Autodesk Inventor part; units mm, degrees
ref_plane "Work Plane2" through (46, 0, 28.75) normal (0.8365, -0.5, 0.2241) x (-0.2588, 0, 0.9659)
ref_plane "YZ Plane" through (0, 0, 0) normal (1, 0, 0) x (0, 1, 0)
ref_plane "XZ Plane" through (0, 0, 0) normal (0, 1, 0) x (-1, 0, 0)
sketch "Sketch1" plane through (0, 0, 0) normal (0, 0, 1) x (1, 0, 0)
  circle A0 centre (0, 0) radius 5
  circle A1 centre (0, 0) radius 8.45
  circle A2 centre (0, 0) radius 42.5
  circle A3 centre (0, 0) radius 45 construction
  circle A4 centre (-31.8198, 31.8198) radius 1.45
  arc A5 (-28.0933, 35.1535) -> (-35.1535, 28.0933) centre (-31.8198, 31.8198) ccw
  arc A6 (-35.1535, -28.0933) -> (-28.0933, -35.1535) centre (-31.8198, -31.8198) ccw
  circle A7 centre (-31.8198, -31.8198) radius 1.45
  arc A8 (28.0933, -35.1535) -> (35.1535, -28.0933) centre (31.8198, -31.8198) ccw
  circle A9 centre (31.8198, -31.8198) radius 1.45
  arc A10 (35.1535, 28.0933) -> (28.0933, 35.1535) centre (31.8198, 31.8198) ccw
  circle A11 centre (31.8198, 31.8198) radius 1.45
  line L0 (-31.8198, 31.8198) -> (31.8198, 31.8198) construction
  arc A12 (28.841, 35.8357) -> (-28.841, 35.8357) centre (0, 0) ccw
  arc A13 (-35.8357, 28.841) -> (-35.8357, -28.841) centre (0, 0) ccw
  arc A14 (-28.841, -35.8357) -> (28.841, -35.8357) centre (0, 0) ccw
  arc A15 (35.8357, -28.841) -> (35.8357, 28.841) centre (0, 0) ccw
  point P0 (0, -46)
  point P1 (0, 46)
  dimension "d2" = 10
  dimension "d3" = 16.9
  dimension "d4" = 85
  dimension "d5" = 90
  dimension "d6" = 2.9
  dimension "d7" = 5
  dimension "d8" = 360
  dimension "d9" = 92
extrude "Extrusion1" add sketch "Sketch1" along normal blind 2.5 contours A1
extrude "Extrusion2" add sketch "Sketch1" along normal blind 7.5 contours A2
extrude "Extrusion3" add sketch "Sketch1" along normal blind 28.75 contours A12 A10 A15 A8 A14 A6 A13 A5
sketch "Sketch2" plane through (0, 0, 28.75) normal (0, 0, 1) x (1, 0, 0)
  arc A0 (35.8357, -28.841) -> (35.8357, 28.841) centre (0, 0) ccw construction
  line L0 (46, 0) -> (46, -31.8198) construction
  point P0 (31.8198, -31.8198)
ref_plane "Work Plane1" through (46, 0, 28.75) normal (0.9659, 0, 0.2588) x (0, -1, 0)
sketch "Sketch3" plane through (46, 0, 28.75) normal (0.9659, 0, 0.2588) x (0, -1, 0)
  ellipse E0 centre (0, -11.9057) end of major axis (-46, -11.9057) minor radius 11.9057 (28.841, -2.6307) -> (-28.841, -2.6307) ccw
  line L0 (0, 0) -> (0, -11.9057) construction
  point P0 (0, 15.8647)
ref_plane "Work Plane2" through (46, 0, 28.75) normal (0.8365, -0.5, 0.2241) x (-0.2588, 0, 0.9659)
sketch "Sketch4" plane through (46, 0, 28.75) normal (0.8365, -0.5, 0.2241) x (-0.2588, 0, 0.9659)
  circle A0 centre (0, 0) radius 5.325
  point P0 (-15.8647, 25.9368)
  dimension "d18" = 10.65
extrude "Extrusion4" cut sketch "Sketch4" along normal mid plane 30
properties part number "Case Part 1 - V2"
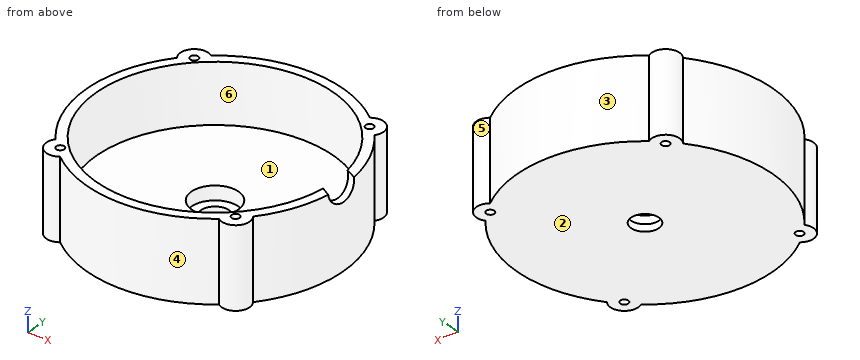
Could you check a few things on this model? Use its own coordinates, in mm. Face numbers are marked on the shaded views. A direction names the side the tool comes from. Give positions to 0.01 mm unless a question says otherwise; leave off trailing zeros. Order: outer loops, then holes, each group sorted by start corner. A loop starts at its lowest first (then second) coordinate and runs counter-clockwise, first axis right, second up.
1. For the marked faces 5 and 6, which set-ups out of +Z, -Z, +X, -X, +Y, -Y let a thin tool reach every point of the face, with its end or its side?
2. We'd pull the mould along Y, two halves only. Please class the marked faces 1, 2, 3 and 4: pulls with the +Y half, pulls with the -Y half, needs draft (parallel to the pull), parting line crosses it, or undercut.
3. I need wall thicknesses on L1, parallel to Y at x = -1, z = 9; L2, parallel to Y at x = 36, z = 19.5. Which ranges of each line are inside material? Lowest first, please.
4. Suppose I cut it at C-C (z = 13.25). List the corners of the cut face in (x, y) for me, plus the area to 3 significant figures.
5. Suppose I cut it at D-D (x = -27). List the corners of the cut face in (y, z) for me.
6. Suppose I cut it at B-B (y = -16.5). List the corners of the cut face in (x, z) for me.
7. Suppose I cut it at A-A (x = 0). List the corners of the cut face in (y, z) for me.
8. Will these pins go through, and if not, where does the flat tip stop? P1, Ø1.7, axis at x = -31.82, y = -31.82, coming from the -Z side; P2, Ø1.5, axis at y = -12, z = 13.5, coming from the +X side; P3, Ø2, axis at y = -28.5, z = 7.5, coming from the -X side; P4, Ø1.5, axis at x = 21.5, z = 22.5, coming from the +Y side.
Solved:
1. face 5: +Z, -Z
1. face 6: +Z
2. face 1: undercut
2. face 2: needs draft
2. face 3: pulls with the +Y half
2. face 4: pulls with the -Y half
3. L1: y = -45.99 to -42.49, 42.49 to 45.99
3. L2: y = -34.56 to -29.08, -28.64 to -22.59, 22.59 to 28.64, 29.08 to 34.56
4. outline: (-35.84, -28.84) arc R5 ccw to (-28.84, -35.84) arc R46 ccw to (28.84, -35.84) arc R5 ccw to (35.84, -28.84) arc R46 ccw to (35.84, 28.84) arc R5 ccw to (28.84, 35.84) arc R46 ccw to (-28.84, 35.84) arc R5 ccw to (-35.84, 28.84) arc R46 ccw to start; hole circle Ø85 at (0, 0); hole circle Ø2.9 at (-31.82, -31.82); hole circle Ø2.9 at (-31.82, 31.82); hole circle Ø2.9 at (31.82, -31.82); hole circle Ø2.9 at (31.82, 31.82)
4. area: 1,070 mm2
5. outline: (-37.24, 0) - (37.24, 0) - (37.24, 28.75) - (32.82, 28.75) - (32.82, 7.5) - (-32.82, 7.5) - (-32.82, 28.75) - (-37.24, 28.75) - close
6. outline: (-42.94, 0) - (42.94, 0) - (42.94, 28.75) - (39.17, 28.75) - (39.17, 7.5) - (-39.17, 7.5) - (-39.17, 28.75) - (-42.94, 28.75) - close
7. outline: (-46, 0) - (-5, 0) - (-5, 2.5) - (-8.45, 2.5) - (-8.45, 7.5) - (-42.5, 7.5) - (-42.5, 28.75) - (-46, 28.75) - close; (5, 0) - (46, 0) - (46, 28.75) - (42.5, 28.75) - (42.5, 7.5) - (8.45, 7.5) - (8.45, 2.5) - (5, 2.5) - close
8. P1: passes through
8. P2: stops at x = 44.6
8. P3: stops at x = -36.87
8. P4: stops at y = 41.05
